```python
from build123d import *

# Parameters (mm, degrees)
SKETCH2_R   = 9.525
SKETCH2_R_2 = 8.2804


with BuildPart() as part:
    # Sweep1: sweep along a path in Sketch1
    with BuildLine(Plane(origin=(0, 0, 0), x_dir=(1, 0, 0), z_dir=(0, 1, 0))) as sweep1_path:
        Line((0, 0), (95.436926547, 0))
        ThreePointArc((95.436926547, 0), (124.597404093, 5.800379623), (149.318463274, 22.318463274))
        Line((149.318463274, 22.318463274), (150.825395518, 23.825395518))
        ThreePointArc((150.825395518, 23.825395518), (175.546454698, 40.343479169), (204.706932244, 46.143858792))
        Line((204.706932244, 46.143858792), (680.250251886, 46.143858792))
        ThreePointArc((680.250251886, 46.143858792), (709.410729432, 40.343479169), (734.131788612, 23.825395518))
        Line((734.131788612, 23.825395518), (803.794862065, -45.837677935))
        ThreePointArc((803.794862065, -45.837677935), (828.515921245, -62.355761586), (857.676398792, -68.156141208))
        Line((857.676398792, -68.156141208), (883.076398792, -68.156141208))
    # Sketch2 → Sweep1 (sweep)
    with BuildSketch(Plane(origin=(0, 0, 0), x_dir=(0, 0, -1), z_dir=(1, 0, 0))):
        Circle(SKETCH2_R)
        Circle(SKETCH2_R_2, mode=Mode.SUBTRACT)
    sweep(path=sweep1_path.line)


solid = part.part
```
For this review, take the finished solid that the model builds, in its own axes (mm). A direction names the side the tool comes from. Coordinates: 2 decimals unless noted, no trailing zeros. Write each loop counter-clockwise with the first axis right and the second up, starting at its lowest first coordinate (ties: lowest second). Pieces come first, ordered by that corner, then holes. Notation, with made-up numbers: (25.5, 88) - (51.5, 88) arc R19 ccw to (51.5, 96) - close; hole circle Ø6 at (13, 63). An arc over 180 degrees is marked (long way). Answer in a Markdown table with one row per item. Add a question column.
Q1. Draft analysis for pull direction Z (two halves, no side actions). For faces 5 (the cylindrical face through (48.387, -5.796, 7.559)), 6 (the cylindrical face through (445.81, 2.49, -54.04)), 7 (the flat face through (883.076, -8, 65)), state which applies: +Z half, -Z half, draft (parallel to the pull), parting line (faces both ways), or undercut.
Q2. For P1, Ø8, axis at x = 751, y = -2.5, coming from the -Z side; P2, Ø2, axis at y = -1.5, z = 43.5, coming from the +X side; P3, Ø10, axis at y = 0, z = -46.14, coming from the +X side, all flat-tipped, find the tip position at first contact; note any pin that passes through.
Q3. We need section A-A, the plane x = 455.5. State the section outline as (y, z) points (3 decimals), and give its area (3 significant figures).
Q4. Tool access review of faces 1 (the flat face through (0, -8, -3)), 2 (the cylindrical face through (48.4, 5.6, 6.1)), 3 (the cylindrical face through (445.81, 2.86, -55.23)), 4 (the cylindrical face through (870.55, 2.86, 59.07)): name each direction out of +Z, -Z, +X, -X, +Y, -Y from which nothing blocks a thin tool from reaching the whole face with its end or side.
Q5. We need section B-B, the plane z = 0. Count the separate pieces of the cut face and the enclosed holes in it, and give its area (3 significant figures).
Q6. For probe 1 along Z at (x, y) = (509, 0); probe 2 along Z at (x, y) = (370, 1); probe 3 along X at (y, z) = (1.25, -44.5), list the stretches that pass through material, from the lowest coordinate up.
Answer list:
| question | item | result |
|---|---|---|
| 1 | face 5 | parting line |
| 1 | face 6 | undercut |
| 1 | face 7 | draft |
| 2 | P1 | stops at z = -24.13 |
| 2 | P2 | stops at x = 816.46 |
| 2 | P3 | stops at x = 728 |
| 3 | outline | circle Ø19.05 at (0, -46.144); hole circle Ø16.561 at (0, -46.144) |
| 3 | area | 69.6 mm2 |
| 4 | face 1 | +Z, -Z, -X, +Y, -Y |
| 4 | face 2 | -X |
| 4 | face 3 | none |
| 4 | face 4 | +X |
| 5 | separate pieces | 2 |
| 5 | enclosed holes | 1 |
| 5 | area | 461 mm2 |
| 6 | probe 1 | z = -55.67 to -54.42, -37.86 to -36.62 |
| 6 | probe 2 | z = -55.62 to -54.36, -37.92 to -36.67 |
| 6 | probe 3 | x = 162.56 to 165.18, 719.78 to 722.39 |
